Model file for the job. Use its own axes, mm. A direction names the side the tool comes from. Round coordinates to 2 decimals unless told otherwise and drop trailing zeros. Loops run counter-clockwise (first coordinate to the right, second up) from the corner with the lowest first, then second, coordinate; pieces in that order, holes last. Notation, with made-up numbers: M 16.5,1 L 58.5,1 A17 cw 58.5,20 Z; hole C -9,31.5 d7. An arc over 180 degrees is marked long. Answer in a Markdown table with one row per item.
from build123d import *

# Parameters (mm, degrees)
SKETCH_R        = 3.6
SKETCH_R_2      = 1.6
SKETCH_W        = 6.5
SKETCH_H        = 3
SKETCH_W_2      = 11.5
PAD_DEPTH       = 9
POCKET_DEPTH    = 2.6
POCKET001_DEPTH = 7
SKETCH003_W     = 25.7
SKETCH003_H     = 13
POCKET002_DEPTH = 3
SKETCH004_R     = 1.8
POCKET003_DEPTH = 2
FILLET_R        = 10
FILLET001_R     = 0.99
FILLET002_R     = 1
FILLET003_R     = 0.5


with BuildPart() as part:
    # Sketch → Pad (new body)
    with BuildSketch(Plane.XY):
        with BuildLine():
            Line((15.5, -31.35), (15.5, -6.75))
            Line((15.5, -6.75), (11.5, -6.75))
            Line((11.5, -6.75), (11.5, 6.75))
            Line((11.5, 6.75), (15.5, 6.75))
            Line((15.5, 6.75), (15.5, 11.85))
            Line((15.5, 11.85), (-15.5, 11.85))
            Line((-15.5, 11.85), (-15.5, -25.7))
            ThreePointArc((-15.5, -25.7), (-14.679899, -27.679899), (-12.7, -28.5))
            Line((-9.7, -28.5), (-12.7, -28.5))
            Line((-9.7, -29.62), (-9.7, -28.5))
            Line((-9.7, -29.62), (7, -29.62))
            Line((7, -29.62), (7, -31.35))
            Line((7, -31.35), (15.5, -31.35))
        make_face()
        Circle(SKETCH_R, mode=Mode.SUBTRACT)
        with Locations((-11, -12.5)):
            Circle(SKETCH_R_2, mode=Mode.SUBTRACT)
        with Locations((11, -12.5)):
            Circle(SKETCH_R_2, mode=Mode.SUBTRACT)
        with Locations((-6, 8.5)):
            Circle(SKETCH_R_2, mode=Mode.SUBTRACT)
        with Locations((8, 8.5)):
            Circle(SKETCH_R_2, mode=Mode.SUBTRACT)
        with Locations((-8.91, -25.81)):
            Rectangle(SKETCH_W, SKETCH_H, mode=Mode.SUBTRACT)
        with Locations((6.35, -25.81)):
            Rectangle(SKETCH_W_2, SKETCH_H, mode=Mode.SUBTRACT)
    extrude(amount=PAD_DEPTH)

    # Sketch001 (on Face28 of Pad) → Pocket (cut)
    with BuildSketch(Plane.XY.offset(9)):
        Polygon((-8.1, -14.174316), (-8.1, -10.825684), (-11, -9.151368), (-13.9, -10.825684), (-13.9, -14.174316), (-11, -15.848632), align=None)
        Polygon((13.9, -14.174316), (13.9, -10.825684), (11, -9.151368), (8.1, -10.825684), (8.1, -14.174316), (11, -15.848632), align=None)
    extrude(amount=-POCKET_DEPTH, mode=Mode.SUBTRACT)

    # Sketch002 → Pocket001 (cut)
    with BuildSketch(Plane(origin=(0, 0, 0), x_dir=(1, 0, 0), z_dir=(0, 0, -1))):
        Polygon((8.25, -4), (6.25, -4), (6.25, -6.25), (-6.25, -6.25), (-6.25, -4), (-8.25, -4), (-8.25, 4), (-6.25, 4), (-6.25, 6.25), (6.25, 6.25), (6.25, 4), (8.25, 4), align=None)
    extrude(amount=-POCKET001_DEPTH, mode=Mode.SUBTRACT)

    # Sketch003 → Pocket002 (cut)
    with BuildSketch(Plane(origin=(0, 0, 0), x_dir=(1, 0, 0), z_dir=(0, 0, -1))):
        with Locations((0, 22)):
            Rectangle(SKETCH003_W, SKETCH003_H)
    extrude(amount=-POCKET002_DEPTH, mode=Mode.SUBTRACT)

    # Sketch004 (on Face57 of Pocket002) → Pocket003 (cut)
    with BuildSketch(Plane(origin=(0, 0, 3), x_dir=(1, 0, 0), z_dir=(0, 0, -1))):
        with Locations((0, 22)):
            Circle(SKETCH004_R)
        with BuildLine():
            Line((1.5, 15.5), (12.85, 15.5))
            Line((12.85, 15.5), (12.85, 20.5))
            Line((12.85, 20.5), (3.5, 20.5))
            ThreePointArc((3.5, 20.5), (2.085786, 19.914214), (1.5, 18.5))
            Line((1.5, 18.5), (1.5, 15.5))
        make_face()
        with BuildLine():
            Line((-1.5, 15.5), (-12.85, 15.5))
            Line((-12.85, 15.5), (-12.85, 20.5))
            Line((-12.85, 20.5), (-3.5, 20.5))
            ThreePointArc((-1.5, 18.5), (-2.085786, 19.914214), (-3.5, 20.5))
            Line((-1.5, 18.5), (-1.5, 15.5))
        make_face()
        with BuildLine():
            Line((12.85, 23.5), (3.5, 23.5))
            ThreePointArc((1.5, 25.5), (2.085786, 24.085786), (3.5, 23.5))
            Line((1.5, 25.5), (1.5, 28.5))
            Line((1.5, 28.5), (12.85, 28.5))
            Line((12.85, 28.5), (12.85, 23.5))
        make_face()
        with BuildLine():
            Line((-12.85, 23.5), (-3.5, 23.5))
            ThreePointArc((-3.5, 23.5), (-2.085786, 24.085786), (-1.5, 25.5))
            Line((-1.5, 25.5), (-1.5, 28.5))
            Line((-1.5, 28.5), (-12.85, 28.5))
            Line((-12.85, 28.5), (-12.85, 23.5))
        make_face()
    extrude(amount=-POCKET003_DEPTH, mode=Mode.SUBTRACT)

    # Fillet
    fillet_edges = [part.edges().sort_by_distance(p)[0] for p in [
        (-15.5, 11.85, 4.5),
    ]]
    fillet(fillet_edges, radius=FILLET_R)

    # Fillet001
    fillet001_edges = [part.edges().sort_by_distance(p)[0] for p in [
        (6.25, -4, 3.5),
        (6.25, -6.25, 3.5),
        (8.25, -4, 3.5),
        (8.25, 4, 3.5),
        (6.25, 4, 3.5),
        (6.25, 6.25, 3.5),
        (-6.25, 6.25, 3.5),
        (-6.25, 4, 3.5),
        (-8.25, 4, 3.5),
        (-8.25, -4, 3.5),
        (-6.25, -4, 3.5),
        (-6.25, -6.25, 3.5),
    ]]
    fillet(fillet001_edges, radius=FILLET001_R)

    # Fillet002
    fillet002_edges = [part.edges().sort_by_distance(p)[0] for p in [
        (15.5, 11.85, 4.5),
        (15.5, -6.75, 4.5),
        (15.5, 6.75, 4.5),
        (15.5, -31.35, 4.5),
        (7, -31.35, 4.5),
        (-9.7, -29.62, 4.5),
        (0.6, -27.31, 6),
        (-12.16, -27.31, 7),
        (-5.66, -27.31, 7),
        (12.1, -27.31, 7),
        (-12.16, -24.31, 7),
        (-5.66, -24.31, 7),
        (12.1, -24.31, 7),
        (0.6, -24.31, 6),
    ]]
    fillet(fillet002_edges, radius=FILLET002_R)

    # Fillet003
    fillet003_edges = [part.edges().sort_by_distance(p)[0] for p in [
        (11.5, 6.75, 4.5),
        (11.5, -6.75, 4.5),
        (7, -29.62, 4.5),
        (12.85, -15.5, 1.5),
        (12.85, -15.5, 4),
        (12.85, -23.5, 4),
        (12.85, -20.5, 4),
        (12.85, -28.5, 1.5),
        (12.85, -28.5, 4),
        (-12.85, -15.5, 1.5),
        (-12.85, -15.5, 4),
        (-12.85, -23.5, 4),
        (-12.85, -20.5, 4),
        (1.5, -27.304987, 4),
        (1.892549, -24.31, 4),
        (-1.8, -22, 5),
    ]]
    fillet(fillet003_edges, radius=FILLET003_R)


solid = part.part
1. Wall check: probe 1 along X at (y, z) = (-12.5, 5.25); probe 2 along X at (y, z) = (-16.5, 3.5); probe 3 along Y at (x, z) = (14, 8.5). Give the ranges that are in metal, low to high.
Verdict:
| item | result |
|---|---|
| probe 1 | x = -15.5 to -12.6, -9.4 to 9.4, 12.6 to 15.5 |
| probe 2 | x = -15.5 to -12.85, -1.5 to 1.5, 12.85 to 15.5 |
| probe 3 | y = -31.35 to -6.75, 6.75 to 11.85 |
2. Mould opens along X. For faces 5 (the flat face through (-11, -28.5, 7)), 6 (the cylindrical face through (-5.95, 5.97, 3.55)), 7 (the flat face through (15.5, 9, 4)) say: +X half, -X half, draft (parallel to the pull), parting line (faces both ways), or undercut.
Verdict:
| item | result |
|---|---|
| face 5 | draft |
| face 6 | undercut |
| face 7 | +X half |
3. Saw through at A-A (y = -12.5). Write the cut outline in (x, z), and give its area (3 significant figures).
Verdict:
| item | result |
|---|---|
| outline | M -15.5,0 L -12.6,0 L -12.6,6.4 L -13.9,6.4 L -13.9,9 L -15.5,9 Z; M -9.4,0 L 9.4,0 L 9.4,6.4 L 8.1,6.4 L 8.1,9 L -8.1,9 L -8.1,6.4 L -9.4,6.4 Z; M 12.6,0 L 15.5,0 L 15.5,9 L 13.9,9 L 13.9,6.4 L 12.6,6.4 Z |
| area | 208 mm² |
4. Pin check, flat tips, straight feed: pin 1 (3.5 mm diameter, centred on x = -11, y = -12.5, fed in from +Z); pin 2 (1 mm diameter, centred on x = -6.5, z = 4, fed in from +Y); pin 3 (4.5 mm diameter, centred on x = 0, y = -22, fed in from -Z). Stop position of each tip, or through.
Verdict:
| item | result |
|---|---|
| pin 1 | stops at z = 6.4 |
| pin 2 | stops at y = 11.84 |
| pin 3 | stops at z = 3 |
5. Saw through at B-B (z = 2.25). State how many separate pieces and enclosed holes the cut face has, and give its area (3 significant figures).
Verdict:
| item | result |
|---|---|
| separate pieces | 1 |
| enclosed holes | 5 |
| area | 662 mm² |
6. Saw through at C-C (y = 4.5). Write the cut outline in (x, z), and give its area (3 significant figures).
Verdict:
| item | result |
|---|---|
| outline | M -15.14,0 L -6.38,0 L -6.38,7 L 6.38,7 L 6.38,0 L 11.5,0 L 11.5,9 L -15.14,9 Z |
| area | 150 mm² |
7. Tool access for faces 1 (the flat face through (8.1, -12, 8)), 2 (the cylindrical face through (-11.859, -27.025, 7.028)), 3 (the cylindrical face through (-6.53, 4.3, 3.55)), 4 (the flat face through (5, 11.85, 4)): list every direction of +Z, -Z, +X, -X, +Y, -Y with a clear straight run to the whole face (end or side of a thin tool).
Verdict:
| item | result |
|---|---|
| face 1 | +Z |
| face 2 | +Z, -Z |
| face 3 | -Z |
| face 4 | +Z, -Z, +X, -X, +Y |
